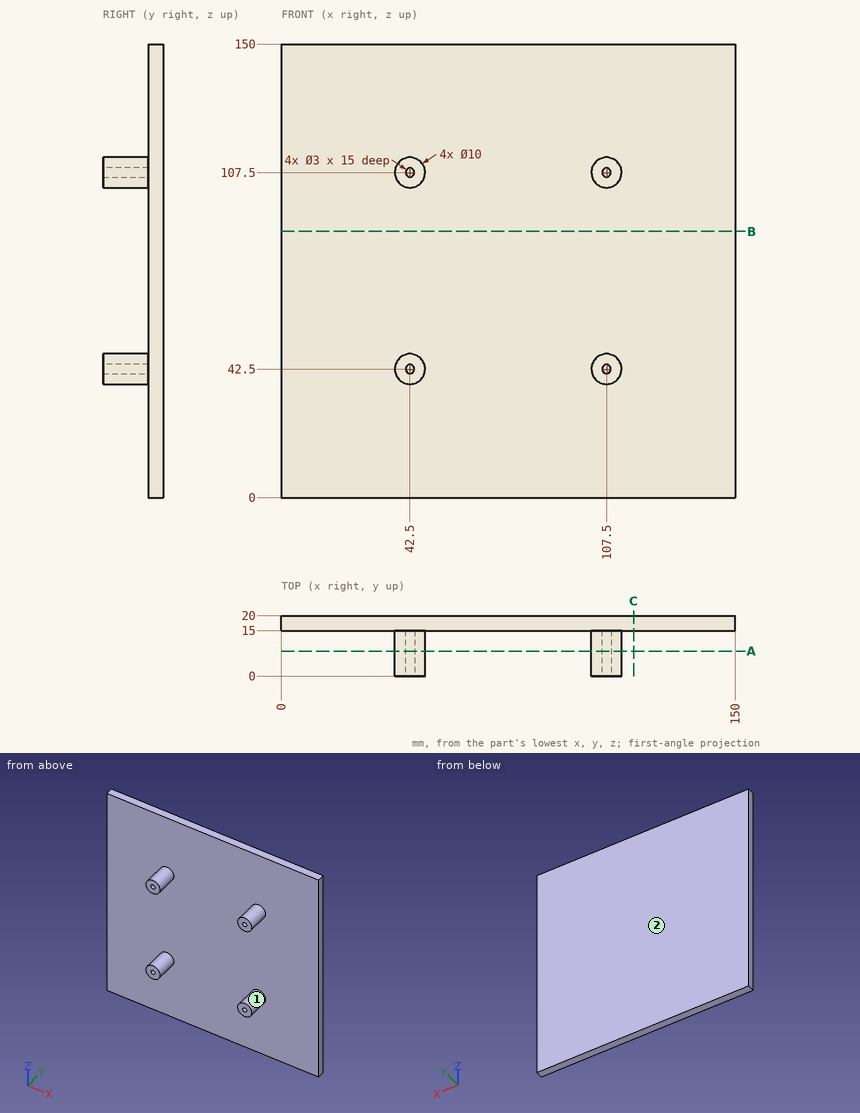
Geometry: see drawing. Coordinates: mm, zero at the bounding-box minimum. Coordinates: 2 decimals unless noted, no trailing zeros. Write each loop counter-clockwise with the first axis right and the second up, starting at its lowest first coordinate (ties: lowest second). Pieces come first, ordered by that corner, then holes.
1) Material intervals for line 1 along X through (y, z) = (8, 42.5); line 2 along Y through (x, z) = (132, 24.5), sorted ascending.
2) Section C-C on x = 116.5. Output: boundary loops of the cut face in (y, z), and give its area (3 significant figures).
3) Section A-A on y = 8.25. Output: boundary loops of the cut face in (x, z), and give its area (3 significant figures).
4) Section B-B on z = 88. Output: boundary loops of the cut face in (x, y).
5) Mould query, pull axis Z, two halves, no side actions, for the marked faces 1 and 2. Classes: pulls with the +Z half, pulls with the -Z half, needs draft (parallel to the pull), parting line crosses it, or undercut.
6) Pin query (flat end, axial travel): pin 1 Ø0.9 at (x, z) = (43, 108) entering from -Y; pin 2 Ø3.5 at (x, z) = (108, 108) entering from -Y; pin 3 Ø12 at (y, z) = (4, 131.5) entering from +X. Return the tip coordinate at first contact, or that it passes through.
Check result:
1. line 1: x = 37.5 to 41, 44 to 47.5, 102.5 to 106, 109 to 112.5
1. line 2: y = 15 to 20
2. outline: (15, 0) - (20, 0) - (20, 150) - (15, 150) - close
2. area: 750 mm2
3. outline: circle Ø10 at (42.5, 42.5); circle Ø10 at (42.5, 107.5); circle Ø10 at (107.5, 42.5); circle Ø10 at (107.5, 107.5); hole circle Ø3 at (42.5, 42.5); hole circle Ø3 at (42.5, 107.5); hole circle Ø3 at (107.5, 42.5); hole circle Ø3 at (107.5, 107.5)
3. area: 286 mm2
4. outline: (0, 15) - (150, 15) - (150, 20) - (0, 20) - close
5. face 1: undercut
5. face 2: needs draft
6. pin 1: stops at y = 15
6. pin 2: stops at y = 0
6. pin 3: passes through
